Autodesk Inventor part; units mm, degrees
ref_plane "Work Plane1" through (0, 0, -15.24) normal (0, 0, -1) x (-1, 0, 0)
ref_plane "YZ Plane" through (0, 0, 0) normal (1, 0, 0) x (0, 1, 0)
ref_plane "XZ Plane" through (0, 0, 0) normal (0, 1, 0) x (-1, 0, 0)
sketch "Sketch1" plane through (0, 0, 0) normal (0, 0, 1) x (1, 0, 0)
  line L0 (33.1238, 20.8366) -> (-2.4362, 20.8366)
  line L1 (-2.4362, 20.8366) -> (-2.4362, -14.7234)
  line L2 (-2.4362, -14.7234) -> (33.1238, -14.7234)
  line L3 (33.1238, -14.7234) -> (33.1238, 20.8366)
  circle A0 centre (4.3476, -7.9396) radius 1.0922
  circle A1 centre (26.34, -7.9396) radius 1.0922
  circle A2 centre (4.3476, 14.0528) radius 1.0922
  circle A3 centre (26.34, 14.0528) radius 1.0922
  line L4 (32.4234, 14.0528) -> (-3.1366, 14.0528) construction
  line L5 (31.7464, -7.9396) -> (-3.8136, -7.9396) construction
  line L6 (4.3476, 22.271) -> (4.3476, -13.289) construction
  line L7 (26.34, 20.1424) -> (26.34, -15.4176) construction
  point P0 (0, 0)
  dimension "CameraHole" = 2.1844
  dimension "BaseWidth" = 35.56
extrude "Base" add sketch "Sketch1" along normal blind 3.81
sketch "Sketch2" plane through (0, 0, 0) normal (0, 0, -1) x (-1, 0, 0)
  line L0 (-12.7595, 17.2806) -> (-17.9281, 17.2806)
  line L1 (-29.5678, 5.6408) -> (-29.5678, 0.4723)
  line L2 (-1.1198, 0.4723) -> (-1.1198, 5.6408)
  line L3 (2.4362, 20.8366) -> (2.4362, -14.7234)
  line L4 (2.4362, -14.7234) -> (-33.1238, -14.7234)
  line L5 (-33.1238, 20.8366) -> (2.4362, 20.8366)
  line L6 (-31.3438, -12.9434) -> (-31.3438, 19.0566) construction
  line L7 (-31.3438, 19.0566) -> (0.6562, 19.0566) construction
  line L8 (0.6562, 19.0566) -> (0.6562, -12.9434) construction
  circle A0 centre (-26.34, 14.0528) radius 1.0922 construction
  line L9 (-1.041, 19.0566) -> (-1.041, 20.8366) construction
  line L10 (-1.1198, 17.2806) -> (-29.5678, 17.2806)
  line L11 (-29.5678, 17.2806) -> (-29.5678, -11.1674)
  line L12 (-17.9281, -11.1674) -> (-12.7595, -11.1674)
  line L13 (-1.1198, -11.1674) -> (-1.1198, 17.2806)
  arc A1 (-26.5198, 10.2967) -> (-22.584, 14.2326) centre (-29.5678, 17.2806) ccw
  arc A2 (-22.584, -8.1194) -> (-26.5198, -4.1836) centre (-29.5678, -11.1674) ccw
  arc A3 (-4.1678, -4.1836) -> (-8.1037, -8.1194) centre (-1.1198, -11.1674) ccw
  arc A4 (-8.1037, 14.2326) -> (-4.1678, 10.2967) centre (-1.1198, 17.2806) ccw
  arc A5 (-29.5678, 0.4723) -> (-26.5198, -4.1836) centre (-24.4878, 0.4723) ccw
  arc A6 (-26.5198, 10.2967) -> (-29.5678, 5.6408) centre (-24.4878, 5.6408) ccw
  arc A7 (-17.9281, 17.2806) -> (-22.584, 14.2326) centre (-17.9281, 12.2006) ccw
  arc A8 (-8.1037, 14.2326) -> (-12.7595, 17.2806) centre (-12.7595, 12.2006) ccw
  arc A9 (-1.1198, 5.6408) -> (-4.1678, 10.2967) centre (-6.1998, 5.6408) ccw
  arc A10 (-4.1678, -4.1836) -> (-1.1198, 0.4723) centre (-6.1998, 0.4723) ccw
  arc A11 (-12.7595, -11.1674) -> (-8.1037, -8.1194) centre (-12.7595, -6.0874) ccw
  arc A12 (-22.584, -8.1194) -> (-17.9281, -11.1674) centre (-17.9281, -6.0874) ccw
  point P0 (-29.5678, 9.6606)
  point P1 (-21.9478, 17.2806)
  point P2 (-21.9478, -11.1674)
  point P3 (-29.5678, -3.5474)
  point P4 (-1.1198, -3.5474)
  point P5 (-8.7398, -11.1674)
  point P6 (-8.7398, 17.2806)
  point P7 (-1.1198, 9.6606)
  dimension "d13" = 3.556
  dimension "d16" = 3.556
  dimension "d38" = 32
  dimension "d101" = 28.448
  dimension "d102" = 7.62
  dimension "d103" = 7.62
  dimension "d104" = 7.62
  dimension "d105" = 7.62
  dimension "d106" = 5.08
extrude "Open Back" cut sketch "Sketch2" against normal blind 3.81 contours A8 A4 A9 L2 A10 A3 A11 L12 A12 A2 A5 L1 A6 A1 A7 L0
sketch "Sketch4" plane through (0, 0, 0) normal (0, 0, -1) x (-1, 0, 0)
  line L0 (-33.1238, 20.8366) -> (2.4362, 20.8366)
  line L1 (2.4362, 20.8366) -> (2.4362, -14.7234)
  line L2 (2.4362, -14.7234) -> (-33.1238, -14.7234)
  line L3 (-33.1238, -14.7234) -> (-33.1238, 20.8366)
  line L4 (1.2932, -13.5804) -> (-31.9808, -13.5804)
  line L5 (-31.9808, -13.5804) -> (-31.9808, 19.6936)
  line L6 (-31.9808, 19.6936) -> (1.2932, 19.6936)
  line L7 (1.2932, 19.6936) -> (1.2932, -13.5804)
  point P0 (0, 0)
  dimension "d32" = 1.143
  dimension "d33" = 1.143
  dimension "d34" = 1.143
  dimension "d35" = 1.143
extrude "Housing" add sketch "Sketch4" along normal blind 15.24
ref_plane "Work Plane1" through (0, 0, -15.24) normal (0, 0, -1) x (-1, 0, 0)
sketch "Sketch10" plane through (0, 0, 3.81) normal (0, 0, 1) x (1, 0, 0)
  circle A0 centre (4.3476, 14.0528) radius 1.0922
  circle A1 centre (4.3476, 14.0528) radius 1.0922
  circle A2 centre (4.3476, -7.9396) radius 1.0922
  circle A3 centre (4.3476, -7.9396) radius 1.0922
  circle A4 centre (26.34, -7.9396) radius 1.0922
  circle A5 centre (26.34, -7.9396) radius 1.0922
  circle A6 centre (26.34, 14.0528) radius 1.0922
  circle A7 centre (26.34, 14.0528) radius 1.0922
  point P0 (0, 0)
extrude "HoleClosing" add sketch "Sketch10" against normal blind 1.27
sketch "Sketch15" plane through (33.1238, -14.7234, 3.81) normal (1, 0, 0) x (0, 0, -1)
  line L0 (3.81, 34.417) -> (19.05, 34.417)
  line L1 (3.81, 34.417) -> (3.81, 1.143)
  line L2 (3.81, 1.143) -> (19.05, 1.143)
  line L3 (19.05, 34.417) -> (19.05, 1.143)
  line L4 (19.05, 34.417) -> (10.16, 34.417)
  line L5 (10.16, 34.417) -> (10.16, 20.193)
  line L6 (13.335, 13.843) -> (3.81, 13.843)
  line L7 (3.81, 13.843) -> (3.81, 26.543)
  line L8 (3.81, 26.543) -> (13.335, 26.543)
  line L9 (10.16, 26.543) -> (13.335, 26.543)
  line L10 (13.335, 26.543) -> (16.51, 20.193)
  line L11 (16.51, 20.193) -> (13.335, 13.843)
  line L12 (10.16, 20.193) -> (3.81, 26.543) construction
  line L13 (10.16, 20.193) -> (3.81, 13.843) construction
  point P0 (3.81, 26.543)
  point P1 (3.81, 13.843)
  dimension "d107" = 8.89
  dimension "d108" = 14.224
extrude "Cable Hole" cut sketch "Sketch15" against normal blind 3.81 contours L8 L10 L11 L6 L1
sketch "Sketch3" plane through (0, 0, 0) normal (0, 0, -1) x (-1, 0, 0)
  circle A0 centre (-4.3476, -7.9396) radius 1.143
  circle A1 centre (-4.3476, -7.9396) radius 2.0805
  circle A2 centre (-4.3476, -7.9396) radius 1.0922
  line L0 (-19.1558, -6.3775) -> (-19.1558, -11.4067)
  circle A3 centre (-4.3476, 14.0528) radius 1.143
  circle A4 centre (-4.3476, 14.0528) radius 2.0828
  circle A5 centre (-4.3476, 14.0528) radius 1.0922
  circle A6 centre (-26.34, 14.0528) radius 2.0828
  circle A7 centre (-26.34, 14.0528) radius 1.143
  circle A8 centre (-26.34, 14.0528) radius 1.0922
  arc A9 (-24.3548, -7.3094) -> (-25.3959, -9.7962) centre (-26.34, -7.9396) ccw
  circle A10 centre (-26.34, -7.9396) radius 1.143
  circle A11 centre (-26.34, -7.9396) radius 1.0922
  circle A12 centre (-26.34, -7.9396) radius 2.0828
  point P0 (0, 0)
  point P1 (-24.3548, -7.3094)
  dimension "d21" = 0.9375
  dimension "d26" = 2.286
  dimension "d30" = 2.286
  dimension "d31" = 0.9398
extrude "Pegs" add sketch "Sketch3" along normal blind 11.5062 contours A1 | A4 | A6 | A12 A9
sketch "Sketch16" plane through (31.9808, -13.5804, -15.24) normal (-1, 0, 0) x (0, 0, 1)
  line L0 (15.24, 3.558) -> (3.7338, 3.558)
  line L1 (15.24, 7.7236) -> (3.7338, 7.7236)
  line L2 (3.7338, 7.7236) -> (3.7338, 3.558)
  line L3 (15.24, 12.7) -> (15.24, 0)
  line L4 (3.7338, 7.7236) -> (15.24, 7.7236)
  line L5 (15.24, 7.7236) -> (15.24, 3.558)
  line L6 (15.24, 3.558) -> (3.7338, 3.558)
  circle A0 centre (10.4775, 5.6408) radius 2.0828
  line L7 (12.065, 10.414) -> (12.065, 6.9891)
  line L8 (12.065, 4.2925) -> (12.065, 0)
  line L9 (15.24, 5.6408) -> (12.5603, 5.6408)
  line L10 (8.3947, 5.6408) -> (3.7338, 5.6408)
  line L11 (10.4775, 10.414) -> (10.4775, 7.7236)
  line L12 (10.4775, 3.558) -> (10.4775, 0)
  line L13 (8.89, 10.414) -> (8.89, 6.9891)
  line L14 (8.89, 4.2925) -> (8.89, 0)
  line L15 (10.4775, 5.6408) -> (10.4775, 27.6372)
  circle A1 centre (10.4775, 27.6372) radius 2.0828
  dimension "d116" = 21.9964
  dimension "d117" = 4.1656
extrude "Zip-Tie Attachment" add sketch "Sketch16" along normal blind 5.6388 contours A1
sketch "Sketch17" plane through (26.34, 14.0528, -11.5062) normal (0, 0, -1) x (-1, 0, 0)
  circle A0 centre (0, 0) radius 1.143
  circle A1 centre (0, 0) radius 1.143
extrude "top left hole" cut sketch "Sketch17" against normal blind 11.5062
equation "\"CameraHole\" = CameraHole_1"
equation "\"BaseWidth\" = BaseWidth_1"
equation "\"d16\" = UsbHoletoWall"
equation "\"BaseWidth_1\" = 35.56"
equation "\"CameraHole_1\" = 2.1844"
equation "\"ZiptieHole\" = 5.08"
equation "\"ZiptieHoletoHoleDistance\" = 2 * ZiptieRadius + WireThickness"
equation "\"WireThickness\" = 4.064"
equation "\"ZiptieRadius\" = 2.54"
equation "\"ZiptieToSide\" = 8.89"
equation "\"UsbHoletoWall\" = 3.556"
equation "\"WasherHolder\" = 12.7"
properties part number "V2_MountHousing_3DPrint"
CAD build for the part. Positions are in the model's coordinates, mm. A direction names the side the tool comes from. Round coordinates to 2 decimals unless told otherwise and drop trailing zeros. Loops run counter-clockwise (first coordinate to the right, second up) from the corner with the lowest first, then second, coordinate; pieces in that order, holes last. Notation, with made-up numbers: (10, 74.5) - (41, 74.5) arc R24 ccw to (41, 90.5) - close; hole circle Ø6 at (5, 11.5). An arc over 180 degrees is marked (long way). Return JSON: item names as keys, results as strings. Group by question number.
Q1. Band-saw the part on A-A on x = 15. Give the cut face in (y, z), plus the area to 3 significant figures.
Q2. Two-plate mould, pull along Y, no slides. Class faces 3 (the face through (15, -14.723, -6)), 4 (the face through (31.981, -1, -11)): +Y half, -Y half, draft (parallel to the pull), parting line (faces both ways), or undercut.
Q3. Band-saw the part on B-B on y = 8.5. Give the cut face in (x, z).
Q4. Tool access for faces 1 (the face through (3, 13, -11.506)), 2 (the face through (6.536, 11.921, 1.878)): list every direction of +Z, -Z, +X, -X, +Y, -Y with a clear straight run to the whole face (end or side of a thin tool).
Q5. Drill centre lines: line 1 along X through (y, z) = (1.5, 0.75); line 2 along Y through (x, z) = (14.5, -1); line 3 along X through (y, z) = (-4.5, -3). Where is each one in solid material? Low to high. Write a range as [from, to].
Q6. Band-saw the part on C-C on y = -3.5. Give the cut face in (x, z), plus the area to 3 significant figures.
Q7. Flat gauge pins, fed straight in: pin 1 Ø0.7 at (x, y) = (26.5, 13.5) entering from -Z; pin 2 Ø4.5 at (x, y) = (27, -9) entering from -Z. Where does each tip first touch, or does it go through?
Q8. Band-saw the part on D-D on y = 1. Give the cut face in (x, z), plus the area to 3 significant figures.
Solutions:
{
 "1": {"outline": "(-14.72, -15.24) - (-13.58, -15.24) - (-13.58, 0) - (-11.17, 0) - (-11.17, 3.81) - (-14.72, 3.81) - close; (17.28, 0) - (19.69, 0) - (19.69, -15.24) - (20.84, -15.24) - (20.84, 3.81) - (17.28, 3.81) - close", "area": "61.9 mm^2"},
 "2": {"face 3": "-Y half", "face 4": "undercut"},
 "3": {"outline": "(-2.44, -15.24) - (-1.29, -15.24) - (-1.29, 0) - (2, 0) - (2, 3.81) - (-2.44, 3.81) - close; (28.69, 0) - (33.12, 0) - (33.12, 3.81) - (28.69, 3.81) - close; (31.98, -15.24) - (33.12, -15.24) - (33.12, -11.18) - (31.98, -11.18) - close"},
 "4": {"face 1": "-Z", "face 2": "+Z, -Z"},
 "5": {"line 1": "x = [-2.44, 1.12], [29.57, 33.12]", "line 2": "y = [-14.72, -13.58], [19.69, 20.84]", "line 3": "x = [-2.44, -1.29], [31.98, 33.12]"},
 "6": {"outline": "(-2.44, -15.24) - (-1.29, -15.24) - (-1.29, 0) - (3.03, 0) - (3.03, 3.81) - (-2.44, 3.81) - close; (27.65, 0) - (31.98, 0) - (31.98, -15.24) - (33.12, -15.24) - (33.12, 3.81) - (27.65, 3.81) - close", "area": "76.5 mm^2"},
 "7": {"pin 1": "stops at z = 2.54", "pin 2": "stops at z = -11.51"},
 "8": {"outline": "(-2.44, -15.24) - (-1.29, -15.24) - (-1.29, 0) - (1.12, 0) - (1.12, 3.81) - (-2.44, 3.81) - close; (29.57, 0) - (33.12, 0) - (33.12, 3.81) - (29.57, 3.81) - close; (31.98, -15.24) - (33.12, -15.24) - (33.12, -10.47) - (31.98, -10.47) - close", "area": "50.0 mm^2"}
}
